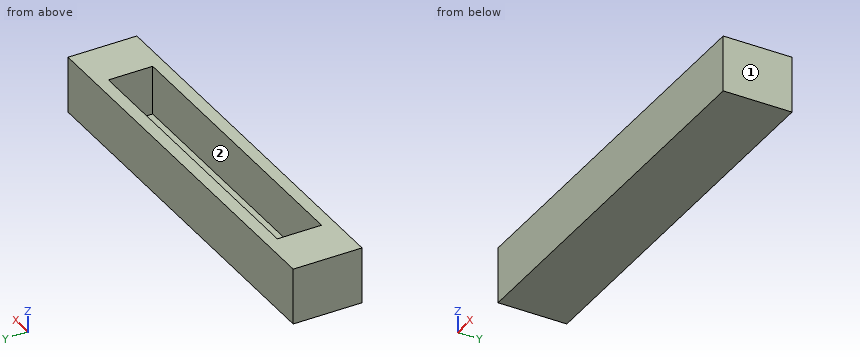
```python
from build123d import *

# Parameters (mm, degrees)
F0_W     = 98
F0_H     = 5
F0_H_2   = 18
F0_W_2   = 11
F1_DEPTH = 3
F2_DEPTH = 23


with BuildPart() as f1:
    # F0 (on Top) → F1 (new body)
    with BuildSketch(Plane.XY):
        Polygon((-80, -14), (-49, -14), (-49, -9), (-60, -9), (-60, 9), (-49, 9), (-49, 14), (-80, 14), align=None)
        with Locations((0, 11.5)):
            Rectangle(F0_W, F0_H)
        Rectangle(F0_W, F0_H_2)
        with Locations((-54.5, 0)):
            Rectangle(F0_W_2, F0_H_2)
        with Locations((0, -11.5)):
            Rectangle(F0_W, F0_H)
        Polygon((49, -14), (80, -14), (80, 14), (49, 14), (49, 9), (60, 9), (60, -9), (49, -9), align=None)
        with Locations((54.5, 0)):
            Rectangle(F0_W_2, F0_H_2)
    extrude(amount=F1_DEPTH)

    # F0 (on Top) → F2 (join)
    with BuildSketch(Plane.XY):
        Polygon((-80, -14), (-49, -14), (-49, -9), (-60, -9), (-60, 9), (-49, 9), (-49, 14), (-80, 14), align=None)
        with Locations((0, 11.5)):
            Rectangle(F0_W, F0_H)
        with Locations((0, -11.5)):
            Rectangle(F0_W, F0_H)
        Polygon((49, -14), (80, -14), (80, 14), (49, 14), (49, 9), (60, 9), (60, -9), (49, -9), align=None)
    extrude(amount=F2_DEPTH)


solid = f1.part
```
The model under review builds one solid part; all positions refer to its coordinate system, in mm. Face numbers are marked on the shaded views. A direction names the side the tool comes from. Round coordinates to 2 decimals unless told otherwise and drop trailing zeros. Loops run counter-clockwise (first coordinate to the right, second up) from the corner with the lowest first, then second, coordinate; pieces in that order, holes last. Notation, with made-up numbers: (57.5, 47.5) -> (92.5, 47.5) arc R20 ccw to (92.5, 81.5) -> close; hole circle Ø10 at (58.5, 68.5). An arc over 180 degrees is marked (long way). Answer in a Markdown table with one row per item.
1) Wall thickness on line 1 along X through (y, z) = (-3.5, 10.5); line 2 along Y through (x, z) = (-6.5, 16.75); line 3 along Z through (x, y) = (36, -7.75): over which ranges is each line inside the solid? List them lowest first.
Taken from the geometry:
| item | result |
|---|---|
| line 1 | x = -80 to -60, 60 to 80 |
| line 2 | y = -14 to -9, 9 to 14 |
| line 3 | z = 0 to 3 |
2) Consider section C-C, the plane x = 13. Write out the cut boundary in (y, z), plus the area to 3 significant figures.
Taken from the geometry:
| item | result |
|---|---|
| outline | (-14, 0) -> (14, 0) -> (14, 23) -> (9, 23) -> (9, 3) -> (-9, 3) -> (-9, 23) -> (-14, 23) -> close |
| area | 284 mm² |
3) Consider section A-A, the plane z = 8.5. Write out the cut boundary in (x, y).
Taken from the geometry:
| item | result |
|---|---|
| outline | (-80, -14) -> (80, -14) -> (80, 14) -> (-80, 14) -> close; hole (-60, -9) -> (60, -9) -> (60, 9) -> (-60, 9) -> close |
4) Consider section B-B, the plane y = 6.25. Write out the cut boundary in (x, z), plus the area to 3 significant figures.
Taken from the geometry:
| item | result |
|---|---|
| outline | (-80, 0) -> (80, 0) -> (80, 23) -> (60, 23) -> (60, 3) -> (-60, 3) -> (-60, 23) -> (-80, 23) -> close |
| area | 1,280 mm² |
5) Tool access review of the marked faces 1 and 2: name each direction out of +Z, -Z, +X, -X, +Y, -Y from which nothing blocks a thin tool from reaching the whole face with its end or side.
Taken from the geometry:
| item | result |
|---|---|
| face 1 | +Z, -Z, +X, +Y, -Y |
| face 2 | +Z |
